Can you work these out from the model? Positions are in its coordinate system, mm. A direction names the side the tool comes from. Coordinates: 2 decimals unless noted, no trailing zeros. Order: outer loops, then holes, each group sorted by start corner. A loop starts at its lowest first (then second) coordinate and runs counter-clockwise, first axis right, second up. Notation, with made-up numbers: (22, -38.5) -> (64, -38.5) arc R12 ccw to (64, -15.5) -> close; hole circle Ø2 at (-1, 46). An arc over 180 degrees is marked (long way). Answer in a Markdown table with one row per item. Add a question column.
1. Will this pin go through, and if not, where does the flat tip stop? pin 1 (1 mm diameter, centred on x = 31, z = 4, fed in from -Y).
2. If I drill on line 1 along Y through (x, z) = (34, 1); line 2 along X through (y, z) = (9.5, 7.25); line 3 along Y through (x, z) = (23, 5.5), over which ranges is the centre line in solid material (lowest first)? Write a range as [from, to].
3. On a 3-axis mill with a long thin cutter (end or side, diameter ignored), from which of +Z, -Z, +X, -X, +Y, -Y can I reach the whole of each face in a straight line? I mean faces 1 (the face through (22, 14.896, 5)), 2 (the face through (0, 24, 5)). Say none if no direction works.
4. We'd pull the mould along Y, two halves only. Please class faces 3 (the face through (36.176, 11, 5)), 4 (the face through (22, 8.082, 5)), 5 (the face through (22, 48.361, 5)), 6 (the face through (22, 25, 10)): pulls with the +Y half, pulls with the -Y half, needs draft (parallel to the pull), parting line crosses it, or undercut.
5. Imagine slicing it at C-C on x = 32. Write out the boundary of the cut face in (y, z), plus the area to 3 significant figures.
6. Imagine slicing it at D-D on z = 9. Write out the boundary of the cut face in (x, y) (3 decimals).
7. Imagine slicing it at A-A on x = 19. Write out the boundary of the cut face in (y, z), plus the area to 3 significant figures.
8. Imagine slicing it at B-B on y = 11. Write out the boundary of the cut face in (x, z).
from build123d import *

# Parameters (mm, degrees)
SKETCH_W      = 44.193939
SKETCH_H      = 48.360676
SKETCH_R      = 6.97501
SKETCH_R_2    = 5.260158
SKETCH_W_2    = 27.894345
SKETCH_H_2    = 6.813885
EXTRUDE_DEPTH = 10


with BuildPart() as part:
    # Sketch → Extrude (new body)
    with BuildSketch(Plane.XY):
        with Locations((22.09697, 24.180338)):
            Rectangle(SKETCH_W, SKETCH_H)
        with Locations((33.621223, 34.272575)):
            Circle(SKETCH_R, mode=Mode.SUBTRACT)
        with Locations((10.837298, 33.953175)):
            Circle(SKETCH_R_2, mode=Mode.SUBTRACT)
        with Locations((22.229264, 11.488646)):
            Rectangle(SKETCH_W_2, SKETCH_H_2, mode=Mode.SUBTRACT)
    extrude(amount=EXTRUDE_DEPTH)


solid = part.part
Answers follow:
| question | item | result |
|---|---|---|
| 1 | pin 1 | stops at y = 0 |
| 2 | line 1 | y = [0, 8.08], [14.9, 27.31], [41.24, 48.36] |
| 2 | line 2 | x = [0, 8.28], [36.18, 44.19] |
| 2 | line 3 | y = [0, 8.08], [14.9, 48.36] |
| 3 | face 1 | +Z, -Z |
| 3 | face 2 | +Z, -Z, -X, +Y, -Y |
| 4 | face 3 | undercut |
| 4 | face 4 | undercut |
| 4 | face 5 | pulls with the +Y half |
| 4 | face 6 | needs draft |
| 5 | outline | (0, 0) -> (8.08, 0) -> (8.08, 10) -> (0, 10) -> close; (14.9, 0) -> (27.49, 0) -> (27.49, 10) -> (14.9, 10) -> close; (41.06, 0) -> (48.36, 0) -> (48.36, 10) -> (41.06, 10) -> close |
| 5 | area | 280 mm² |
| 6 | outline | (0, 0) -> (44.194, 0) -> (44.194, 48.361) -> (0, 48.361) -> close; hole circle Ø10.52 at (10.837, 33.953); hole (8.282, 8.082) -> (36.176, 8.082) -> (36.176, 14.896) -> (8.282, 14.896) -> close; hole circle Ø13.95 at (33.621, 34.273) |
| 7 | outline | (0, 0) -> (8.08, 0) -> (8.08, 10) -> (0, 10) -> close; (14.9, 0) -> (48.36, 0) -> (48.36, 10) -> (14.9, 10) -> close |
| 7 | area | 415 mm² |
| 8 | outline | (0, 0) -> (8.28, 0) -> (8.28, 10) -> (0, 10) -> close; (36.18, 0) -> (44.19, 0) -> (44.19, 10) -> (36.18, 10) -> close |
